Verification items for the finished model (mm, model axes). Face numbers are marked on the shaded views. A direction names the side the tool comes from. Give positions to 0.01 mm unless a question says otherwise; leave off trailing zeros. Loops run counter-clockwise (first coordinate to the right, second up) from the corner with the lowest first, then second, coordinate; pieces in that order, holes last. Notation, with made-up numbers: (83.5, 60) - (121.5, 60) arc R19 ccw to (121.5, 89) - close; hole circle Ø8 at (-25, -24). An arc over 180 degrees is marked (long way). Answer in a Markdown table with one row per item.
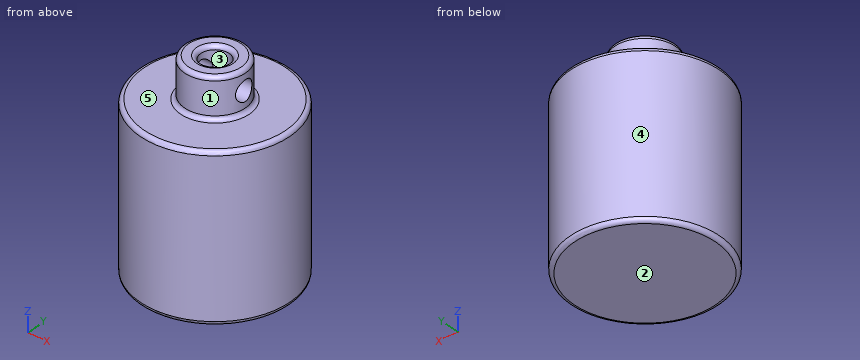
```python
from build123d import *

# Parameters (mm, degrees)
SKETCH1_R           = 18.5
BOSS_EXTRUDE1_DEPTH = 40
SKETCH2_R           = 7.5
BOSS_EXTRUDE2_DEPTH = 10
SKETCH3_R           = 3.5
CUT_EXTRUDE1_DEPTH  = 32
FILLET1_R           = 1
FILLET2_R           = 1
FILLET3_R           = 1
FILLET4_R           = 1
FILLET6_R           = 1
SKETCH4_R           = 2.5
CUT_EXTRUDE2_DEPTH  = 141


with BuildPart() as part:
    # Sketch1 → Boss-Extrude1 (new body)
    with BuildSketch(Plane.XY):
        Circle(SKETCH1_R)
    extrude(amount=BOSS_EXTRUDE1_DEPTH)

    # Sketch2 → Boss-Extrude2 (add)
    with BuildSketch(Plane.XY.offset(40)):
        Circle(SKETCH2_R)
    extrude(amount=BOSS_EXTRUDE2_DEPTH)

    # Sketch3 → Cut-Extrude1 (cut)
    with BuildSketch(Plane.XY.offset(50)):
        Circle(SKETCH3_R)
    extrude(amount=-CUT_EXTRUDE1_DEPTH, mode=Mode.SUBTRACT)

    # Fillet1
    fillet1_edges = [part.edges().sort_by_distance(p)[0] for p in [
        (-7.5, 0, 50),
    ]]
    fillet(fillet1_edges, radius=FILLET1_R)

    # Fillet2
    fillet2_edges = [part.edges().sort_by_distance(p)[0] for p in [
        (-18.5, 0, 40),
    ]]
    fillet(fillet2_edges, radius=FILLET2_R)

    # Fillet3
    fillet3_edges = [part.edges().sort_by_distance(p)[0] for p in [
        (-7.5, 0, 40),
    ]]
    fillet(fillet3_edges, radius=FILLET3_R)

    # Fillet4
    fillet4_edges = [part.edges().sort_by_distance(p)[0] for p in [
        (-18.5, 0, 0),
    ]]
    fillet(fillet4_edges, radius=FILLET4_R)

    # Fillet6
    fillet6_edges = [part.edges().sort_by_distance(p)[0] for p in [
        (-3.5, 0, 50),
    ]]
    fillet(fillet6_edges, radius=FILLET6_R)

    # Sketch4 → Cut-Extrude2 (cut, symmetric)
    with BuildSketch(Plane(origin=(0, 0, 0), x_dir=(0, 0, -1), z_dir=(1, 0, 0))):
        with Locations((-45, 0)):
            Circle(SKETCH4_R)
    extrude(amount=CUT_EXTRUDE2_DEPTH, both=True, mode=Mode.SUBTRACT)


solid = part.part
```
Q1. Sectioned sample at B-B (x = 0). Record the cut outline in (y, z), and give its area (3 significant figures).
Completed:
| item | result |
|---|---|
| outline | (-18.5, 1) arc R1 ccw to (-17.5, 0) - (17.5, 0) arc R1 ccw to (18.5, 1) - (18.5, 39) arc R1 ccw to (17.5, 40) - (8.5, 40) arc R1 cw to (7.5, 41) - (7.5, 49) arc R1 ccw to (6.5, 50) - (4.5, 50) arc R1 ccw to (3.5, 49) - (3.5, 18) - (-3.5, 18) - (-3.5, 49) arc R1 ccw to (-4.5, 50) - (-6.5, 50) arc R1 ccw to (-7.5, 49) - (-7.5, 41) arc R1 cw to (-8.5, 40) - (-17.5, 40) arc R1 ccw to (-18.5, 39) - close |
| area | 1,400 mm^2 |
Q2. Sectioned sample at C-C (z = 33.5). Record the cut outline in (x, y).
Completed:
| item | result |
|---|---|
| outline | circle Ø37 at (0, 0); hole circle Ø7 at (0, 0) |
Q3. Sectioned sample at A-A (y = 0). Give the number of separate pieces and of enclosed holes in the cut face, and give its area (3 significant figures).
Completed:
| item | result |
|---|---|
| separate pieces | 3 |
| enclosed holes | 0 |
| area | 1,360 mm^2 |
Q4. Draft check along X on the marked faces 3, 4 and 5. Enter one of: +X half, -X half, draft (parallel to the pull), parting line (faces both ways), or undercut.
Completed:
| item | result |
|---|---|
| face 3 | undercut |
| face 4 | parting line |
| face 5 | draft |
Q5. Tool access check on the marked faces 1 and 2. Record the directions out of +Z, -Z, +X, -X, +Y, -Y that give a thin tool (end or side, any length) a straight path to the whole face; none if there is none.
Completed:
| item | result |
|---|---|
| face 1 | +Z |
| face 2 | -Z, +X, -X, +Y, -Y |
Q6. Go/stop test with flat-tipped pins: P1, Ø1.5, axis at x = 1.5, z = 5, coming from the +Y side; P2, Ø4, axis at x = -10.5, z = 24.5, coming from the -Y side; P3, Ø1, axis at x = -2, z = 43, coming from the +Y side. Record where each tip stops, or that it passes through.
Completed:
| item | result |
|---|---|
| P1 | y = 18.48 |
| P2 | y = -16.43 |
| P3 | y = 7.35 |
Q7. Sectioned sample at D-D (z = 45). Record the cut outline in (x, y), and give its area (3 significant figures).
Completed:
| item | result |
|---|---|
| outline | (-7.07, -2.5) arc R7.5 ccw to (7.07, -2.5) - (2.45, -2.5) arc R3.5 cw to (-2.45, -2.5) - close; (-7.07, 2.5) - (-2.45, 2.5) arc R3.5 cw to (2.45, 2.5) - (7.07, 2.5) arc R7.5 ccw to start |
| area | 96.4 mm^2 |
Q8. Thickness scan on line 1 (Y direction, x = 0, z = 27); line 2 (Y direction, x = 0, z = 41); line 3 (Z direction, x = 1, y = -16). Record the ranges inside material, lowest first.
Completed:
| item | result |
|---|---|
| line 1 | -18.5 to -3.5, 3.5 to 18.5 |
| line 2 | -7.5 to -3.5, 3.5 to 7.5 |
| line 3 | 0 to 40 |
